```python
from build123d import *

# Parameters (mm, degrees)
BOSS_EXTRUDE1_DEPTH = 6
SKETCH2_W           = 6
SKETCH2_H           = 225
CUT_EXTRUDE1_DEPTH  = 6
LPATTERN1_COUNT     = 2
LPATTERN1_PITCH     = 424


with BuildPart() as part:
    # Sketch1 → Boss-Extrude1 (new body)
    with BuildSketch(Plane(origin=(0, 0, 0), x_dir=(1, 0, 0), z_dir=(0, 1, 0))):
        Polygon((-470, 0), (-430, 0), (-430, 6), (-255, 6), (-255, 0), (-215, 0), (-215, 6), (-40, 6), (-40, 0), (0, 0), (0, 456), (-470, 456), align=None)
    extrude(amount=BOSS_EXTRUDE1_DEPTH)

    # Sketch2 → Cut-Extrude1 (cut)
    with BuildSketch(Plane(origin=(0, 6, 0), x_dir=(1, 0, 0), z_dir=(0, 1, 0))):
        with Locations((-13, 343.5)):
            Rectangle(SKETCH2_W, SKETCH2_H)
    cut_extrude1 = extrude(amount=-CUT_EXTRUDE1_DEPTH, mode=Mode.SUBTRACT)

    # LPattern1: Cut-Extrude1 ×2
    with Locations(*[(-i * LPATTERN1_PITCH, 0, 0) for i in range(1, LPATTERN1_COUNT)]):
        add(cut_extrude1, mode=Mode.SUBTRACT)


solid = part.part
```
Part model, mm, in its own coordinate system. Give positions to 0.01 mm unless a question says otherwise; leave off trailing zeros. Order: outer loops, then holes, each group sorted by start corner. A loop starts at its lowest first (then second) coordinate and runs counter-clockwise, first axis right, second up. Notation, with made-up numbers: (30, -6) - (44, -6) arc R20 cw to (44, 29) - close; hole circle Ø8 at (71.5, 81). An arc over 180 degrees is marked (long way). Use one line per item in the form item = value.
Item 1: Pin check, flat tips, straight feed: pin 1 Ø3 at (x, z) = (-384.5, -367) entering from -Y; pin 2 Ø3 at (x, y) = (-12.5, 3.5) entering from -Z. Stop position of each tip, or through.
Solution:
pin_1 = 0
pin_2 = -231
Item 2: Slice it at A-A on z = -333. Give the cut face in (x, y), and give its area (3 significant figures).
Solution:
outline = (-470, 0) - (-440, 0) - (-440, 6) - (-470, 6) - close; (-434, 0) - (-16, 0) - (-16, 6) - (-434, 6) - close; (-10, 0) - (0, 0) - (0, 6) - (-10, 6) - close
area = 2,750 mm2
Item 3: Probe probe 1 along X at (y, z) = (3.2, -421.5); probe 2 along Z at (x, y) = (-194.5, 3.2). List the from-to ranges inside material, lowest first. Write a range as from..to.
Solution:
probe_1 = -470..-440, -434..-16, -10..0
probe_2 = -456..-6
Item 4: Slice it at B-B on y = 3.95. Give the cut face in (x, z), and give its area (3 significant figures).
Solution:
outline = (-470, -456) - (-440, -456) - (-440, -231) - (-434, -231) - (-434, -456) - (-16, -456) - (-16, -231) - (-10, -231) - (-10, -456) - (0, -456) - (0, 0) - (-40, 0) - (-40, -6) - (-215, -6) - (-215, 0) - (-255, 0) - (-255, -6) - (-430, -6) - (-430, 0) - (-470, 0) - close
area = 210,000 mm2
